Check sheet for the modelled part. Datum: model origin and axes. Units: mm. Face numbers are marked on the shaded views. A direction names the side the tool comes from. Coordinates: 2 decimals unless noted, no trailing zeros. Order: outer loops, then holes, each group sorted by start corner. A loop starts at its lowest first (then second) coordinate and runs counter-clockwise, first axis right, second up.
1. Cross-section at B-B (z = -4.5). Enter the section's corners in (x, y), then the cut area to 3 significant figures.
2. Cross-section at A-A (y = 21). Enter the section's corners in (x, z).
3. Cross-section at D-D (x = 0). Enter the section's corners in (y, z).
4. Cross-section at C-C (y = 9.18). Enter the section's corners in (x, z).
5. Set-up check for the marked faces 1 and 2: record each of +Z, -Z, +X, -X, +Y, -Y from which the full face is reachable in a straight line by a thin tool's end or side.
6. Thickness scan on line 1 (X direction, y = 29.7, z = -19.65); line 2 (X direction, y = 1.15, z = 9.5); line 3 (Z direction, x = -9, y = 11). Record the ranges inside material, lowest first.
7. Gauge pin test, flat ends, axial feed: pin 1 Ø6 at (x, z) = (5, 3.5) entering from +Y; pin 2 Ø1.9 at (x, y) = (0, 9.18) entering from -Z; pin 3 Ø2.5 at (x, z) = (7, -4.5) entering from +Y; pin 4 Ø0.8 at (x, z) = (8, -19) entering from +Y. Record the tip position at first contact, or that the pin passes through.
8. Draft check along Z on the marked faces 3, 4 and 5. Enter one of: released by +Z, released by -Z, zero draft, split by the parting line, or undercut.
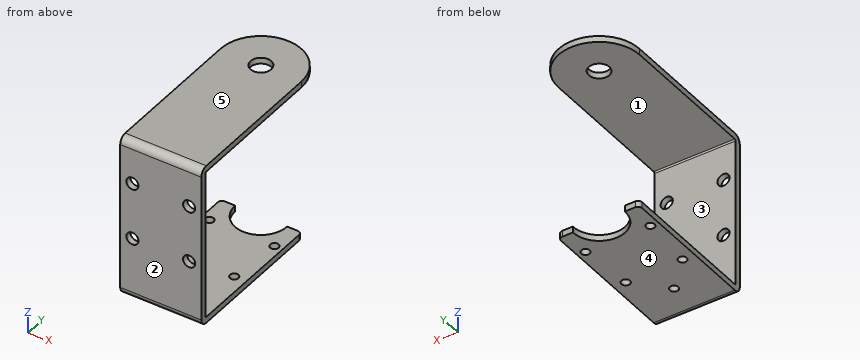
Autodesk Inventor part; units mm, degrees
ref_plane "YZ Plane" through (0, 0, 0) normal (1, 0, 0) x (0, 1, 0)
ref_plane "XZ Plane" through (0, 0, 0) normal (0, 1, 0) x (-1, 0, 0)
ref_plane "XY Plane" through (0, 0, 0) normal (0, 0, 1) x (1, 0, 0)
sketch "Sketch1" plane through (0, 0, 0) normal (0, 1, 0) x (-1, 0, 0)
  line L0 (10, -18.5) -> (-10, -18.5)
  line L1 (-10, -18.5) -> (-10, 18.5)
  line L2 (-10, 18.5) -> (10, 18.5)
  line L3 (10, 18.5) -> (10, -18.5)
  point P0 (0, 0)
  dimension "d0" = 20
  dimension "d1" = 37
  dimension "d2" = 18.5
  dimension "d3" = 10
extrude "Plate1" add sketch "Sketch1" along normal blind 1.5
sketch "Sketch2" plane through (-10, 0, -20) normal (0, 0, 1) x (1, 0, 0)
  line L0 (20, 0) -> (0, 0)
  line L1 (0, 0) -> (0, 46.6)
  line L2 (0, 46.6) -> (20, 46.6)
  line L3 (20, 46.6) -> (20, 0)
edge flange "Flange1" height 46.6 angle 90 thickness 1.5 bend radius 0.31 thickness toward (0, 0, 1) relief tear relief width 1.5 relief depth 0.75 edges at (0, 1.5, -18.5) wall of the first edge with corners at (10, 0, -20) (-10, 0, -20) (-10, 46.6, -20) (10, 46.6, -20)
bend "Bend1"
corner "Corner1"
sketch "Sketch3" plane through (10, 0, 20) normal (0, 0, -1) x (-1, 0, 0)
  line L0 (20, 0) -> (0, 0)
  line L1 (0, 0) -> (0, 46.6)
  line L2 (0, 46.6) -> (20, 46.6)
  line L3 (20, 46.6) -> (20, 0)
edge flange "Flange2" height 46.6 angle 90 thickness 1.5 bend radius 0.31 thickness toward (0, 0, -1) relief tear relief width 1.5 relief depth 0.75 edges at (0, 1.5, 18.5) wall of the first edge with corners at (-10, 0, 20) (10, 0, 20) (10, 46.6, 20) (-10, 46.6, 20)
bend "Bend2"
corner "Corner2"
sketch "Sketch4" plane through (-10, 46.6, 20) normal (0, 0, 1) x (1, 0, 0)
  circle A0 centre (10, -10) radius 10
  line L0 (0, 0) -> (20, 0)
  line L1 (0, 0) -> (20, 0)
  line L2 (20, 0) -> (20, -10)
  line L3 (20, -10) -> (0, -10)
  line L4 (0, -10) -> (0, 0)
  line L5 (0, -44.79) -> (0, 0)
  point P0 (10, -46.6)
  point P1 (10, -10)
  point P2 (20, 0)
  point P3 (10, 0)
  point P4 (0, -10)
  point P5 (8.5893, 0)
  point P6 (0, -10)
  dimension "d26" = 20
  dimension "d25" = 10
  dimension "d27" = 10
  dimension "d28" = 10
extrude "Extrusion1" cut sketch "Sketch4" against normal blind 10 contours L4 L0 A0 | A0 L0 L2
sketch "Sketch5" plane through (10, 46.6, -20) normal (0, 0, -1) x (-1, 0, 0)
  arc A0 (20, -10) -> (0, -10) centre (10, -10) ccw
  point P0 (10, -46.6)
hole "Hole1" at (0, 36.6, -20) direction (0, 0, 1) diameter 12.8 depth 1.5
sketch "Sketch6" plane through (10, 46.6, -20) normal (0, 0, -1) x (-1, 0, 0)
  circle A0 centre (10, -10) radius 6.4
  line L0 (0, 0) -> (20, 0)
  line L1 (0, -44.79) -> (0, 0)
  line L2 (24, 0) -> (-4, 0)
  line L3 (-4, 0) -> (-4, -9.9)
  line L4 (-4, -9.9) -> (24, -9.9)
  line L5 (24, -9.9) -> (24, 0)
  point P0 (10, -46.6)
  point P1 (20, 0)
  point P2 (6.005, 0)
  point P3 (13.995, 0)
  dimension "d38" = 9.9
  dimension "d39" = 4
  dimension "d40" = 28
extrude "Extrusion2" cut sketch "Sketch6" against normal blind 10 contours L4 A0 | A0 L4 L1 L0 L2 L5 | L4 L3 L2 L1 picked at (9.1972, -6.4205)
fillet "Fillet1" radius 1 2 edges at (-10, 36.7, -19.25) (10, 36.7, -19.25)
sketch "Sketch7" plane through (-10, 1.81, 20) normal (0, 0, 1) x (1, 0, 0)
  arc A0 (20, 34.79) -> (0, 34.79) centre (10, 34.79) ccw
  point P0 (10, -1.81)
hole "Hole2" at (0, 36.6, 20) direction (0, 0, -1) diameter 5.1 depth 1.5
sketch "Sketch8" plane through (0, 0, 0) normal (0, -1, 0) x (1, 0, 0)
  line L0 (2.55, 18.5) -> (-2.55, 18.5)
  line L1 (-10, 18.5) -> (10, 18.5)
  line L2 (10, 18.5) -> (-10, 18.5)
  line L3 (10, 18.19) -> (-10, 18.19)
  line L4 (-10, -18.19) -> (-10, 18.19)
  line L5 (-10, -18.19) -> (10, -18.19)
  line L6 (10, 18.19) -> (10, -18.19)
  point P0 (0, 0)
  point P1 (7, 9.5)
  point P2 (7, -4.5)
  point P3 (-7, 9.5)
  point P4 (-7, -4.5)
  dimension "d51" = 9
  dimension "d52" = 3
  dimension "d55" = 14
  dimension "d58" = 14
hole "Hole3" at (7, 0, 9.5) at (7, 0, -4.5) at (-7, 0, 9.5) at (-7, 0, -4.5) direction (0, 1, 0) diameter 3 depth 1.5
hole "Hole5" at (-8, 29.7, -18.5) at (8, 29.7, -18.5) at (7, 16.48, -18.5) at (-7, 16.48, -18.5) at (0, 9.18, -18.5) direction (0, 0, -1) diameter 2.1 depth 1.5
equation "\"d36\" = Thickness"
equation "\"d49\" = Thickness"
equation "\"d66\" = Thickness"
equation "\"d80\" = Thickness"
equation "\"d4\" = Thickness"
equation "\"d5\" = BendReliefWidth"
equation "\"d6\" = BendReliefDepth"
equation "\"d7\" = MinimumRemnant"
equation "\"d8\" = TransitionRadius"
equation "\"d11\" = BendRadius"
equation "\"d12\" = CornerReliefSize"
equation "\"d13\" = GapSize"
equation "\"d14\" = JacobiRadiusSize"
equation "\"d15\" = BendReliefWidth"
equation "\"d16\" = BendReliefDepth"
equation "\"d17\" = MinimumRemnant"
equation "\"d18\" = TransitionRadius"
equation "\"d21\" = BendRadius"
equation "\"d22\" = CornerReliefSize"
equation "\"d23\" = GapSize"
equation "\"d24\" = JacobiRadiusSize"
equation "\"BendReliefWidth\" = Thickness"
equation "\"BendReliefDepth\" = 0.5 * Thickness"
equation "\"CornerReliefSize\" = 4 * Thickness"
equation "\"MinimumRemnant\" = 2 * Thickness"
equation "\"TransitionRadius\" = BendRadius"
equation "\"JacobiRadiusSize\" = BendRadius"
equation "\"GapSize\" = Thickness"
properties part number "axis_9_bottom_frame" material "Aluminum 6061-AHC"
Data:
1. outline: (-10, 0) - (-8.5, 0) - (-8.5, 1.5) - (-10, 1.5) - close; (-5.5, 0) - (5.5, 0) - (5.5, 1.5) - (-5.5, 1.5) - close; (8.5, 0) - (10, 0) - (10, 1.5) - (8.5, 1.5) - close
1. area: 21.0 mm2
2. outline: (-10, -20) - (10, -20) - (10, -18.5) - (-10, -18.5) - close; (-10, 18.5) - (10, 18.5) - (10, 20) - (-10, 20) - close
3. outline: (0, -18.19) arc R1.81 ccw to (1.81, -20) - (8.13, -20) - (8.13, -18.5) - (1.81, -18.5) arc R0.31 cw to (1.5, -18.19) - (1.5, 18.19) arc R0.31 cw to (1.81, 18.5) - (34.05, 18.5) - (34.05, 20) - (1.81, 20) arc R1.81 ccw to (0, 18.19) - close; (10.23, -20) - (30.2, -20) - (30.2, -18.5) - (10.23, -18.5) - close; (39.15, 18.5) - (46.6, 18.5) - (46.6, 20) - (39.15, 20) - close
4. outline: (-10, -20) - (-1.05, -20) - (-1.05, -18.5) - (-10, -18.5) - close; (-10, 18.5) - (10, 18.5) - (10, 20) - (-10, 20) - close; (1.05, -20) - (10, -20) - (10, -18.5) - (1.05, -18.5) - close
5. face 1: +X, -X, +Y
5. face 2: +Z, -Z, +X, -X, -Y
6. line 1: x = -10 to -9.05, -6.95 to 6.95, 9.05 to 10
6. line 2: x = -10 to -8.5, -5.5 to 5.5, 8.5 to 10
6. line 3: z = -20 to -18.5, 18.5 to 20
7. pin 1: stops at y = 1.5
7. pin 2: stops at z = 18.5
7. pin 3: passes through
7. pin 4: stops at y = 36.7
8. face 3: undercut
8. face 4: released by -Z
8. face 5: released by +Z
